Work out the finished part from the listing and answer in its coordinate system (mm). Face numbers are marked on the shaded views. Coordinates: 2 decimals unless noted, no trailing zeros. Order: outer loops, then holes, each group sorted by start corner. A loop starts at its lowest first (then second) coordinate and runs counter-clockwise, first axis right, second up. Notation, with made-up numbers: M 29.5,40.25 L 61.5,40.25 A20 cw 61.5,60.25 Z; hole C 40.5,54 d1. An arc over 180 degrees is marked long. Answer in a Markdown table with one row per item. Add a question column.
Item 1: Flat-ended cylindrical pins translate along their axes: pin 1 Ø3 at (x, y) = (42.5, 19.5) entering from +Z; pin 2 Ø1 at (x, z) = (43.5, -2) entering from -Y; pin 3 Ø1.6 at (y, z) = (32, -2) entering from +X; pin 4 Ø1 at (y, z) = (7.5, -0.5) entering from +X. Find the tip coordinate at first contact, or state that the pin passes through.
Item 2: Consider line 1 (Y direction, x = 12.7, z = -1.5); line 2 (Y direction, x = 14, z = -2.35); line 3 (X direction, y = 39.5, z = -0.75). Determine where each line is inside the solid, lowest interval first. Write a range as from..to.
Item 3: The part is cut by section B-B (y = 63.5). Write down the section's boundary in (x, z) (3 decimals).
Item 4: The part is cut by section C-C (y = 12.7). Write down the section's boundary in (x, z) (3 decimals), then the cut area to 3 significant figures.
Item 5: The mould has two halves that part along Z. Classify the marked faces 1 and 2: released by +Z, released by -Z, zero draft, split by the parting line, or undercut.
Item 6: The part is cut by section A-A (x = 63.5). Write down the section's boundary in (y, z) (3 decimals).
Item 7: The part is cut by section D-D (z = -1.1). Write down the section's boundary in (x, y).
from build123d import *

# Parameters (mm, degrees)
BOSS_EXTRUDE1_DEPTH = 3.175
SKETCH2_R           = 2.4892
CUT_EXTRUDE1_DEPTH  = 108.809835474
FILLET3_R           = 2.54


with BuildPart() as part:
    # Sketch1 → Boss-Extrude1 (new body)
    with BuildSketch(Plane.XY):
        Polygon((25.4, 0), (0, 0), (0, 76.2), (76.2, 76.2), (76.2, 50.8), align=None)
        Polygon((58.239487758, 50.8), (25.4, 50.8), (25.4, 17.960512242), align=None, mode=Mode.SUBTRACT)
    extrude(amount=-BOSS_EXTRUDE1_DEPTH)

    # Sketch2 → Cut-Extrude1 (cut, through all)
    with BuildSketch(Plane.XY):
        with Locations((12.7, 63.5)):
            Circle(SKETCH2_R)
        with Locations((38.1, 63.5)):
            Circle(SKETCH2_R)
        with Locations((63.5, 63.5)):
            Circle(SKETCH2_R)
        with Locations((12.7, 38.1)):
            Circle(SKETCH2_R)
        with Locations((12.7, 12.7)):
            Circle(SKETCH2_R)
    extrude(amount=-CUT_EXTRUDE1_DEPTH, mode=Mode.SUBTRACT)

    # Fillet3
    fillet3_edges = [part.edges().sort_by_distance(p)[0] for p in [
        (25.4, 50.8, -1.5875),
        (25.4, 17.960512242, -1.5875),
        (58.239487758, 50.8, -1.5875),
        (0, 0, -1.5875),
        (0, 76.2, -1.5875),
        (76.2, 76.2, -1.5875),
        (76.2, 50.8, -1.5875),
        (25.4, 0, -1.5875),
    ]]
    fillet(fillet3_edges, radius=FILLET3_R)


solid = part.part
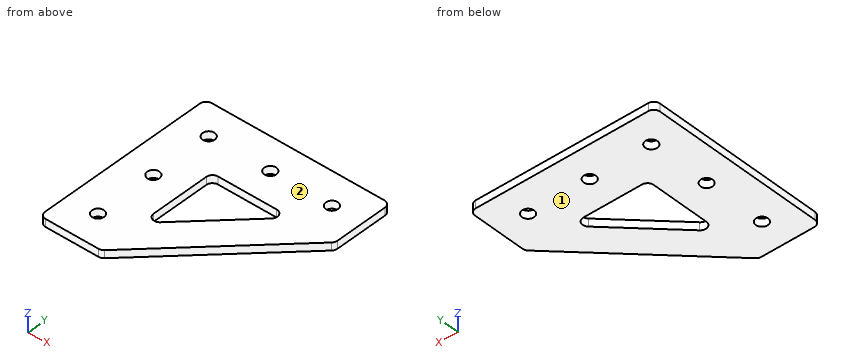
Reply:
| question | item | result |
|---|---|---|
| 1 | pin 1 | stops at z = 0 |
| 1 | pin 2 | stops at y = 17.6 |
| 1 | pin 3 | stops at x = 58.2 |
| 1 | pin 4 | stops at x = 33.4 |
| 2 | line 1 | y = 0..10.21, 15.19..35.61, 40.59..61.01, 65.99..76.2 |
| 2 | line 2 | y = 0..10.58, 14.82..35.98, 40.22..61.38, 65.62..76.2 |
| 2 | line 3 | x = 0..10.64, 14.76..25.4, 46.94..64.9 |
| 3 | outline | M 0,-3.175 L 10.211,-3.175 L 10.211,0 L 0,0 Z; M 15.189,-3.175 L 35.611,-3.175 L 35.611,0 L 15.189,0 Z; M 40.589,-3.175 L 61.011,-3.175 L 61.011,0 L 40.589,0 Z; M 65.989,-3.175 L 76.2,-3.175 L 76.2,0 L 65.989,0 Z |
| 4 | outline | M 0,-3.175 L 10.211,-3.175 L 10.211,0 L 0,0 Z; M 15.189,-3.175 L 38.1,-3.175 L 38.1,0 L 15.189,0 Z |
| 4 | area | 105 mm2 |
| 5 | face 1 | released by -Z |
| 5 | face 2 | released by +Z |
| 6 | outline | M 38.1,-3.175 L 61.011,-3.175 L 61.011,0 L 38.1,0 Z; M 65.989,-3.175 L 76.2,-3.175 L 76.2,0 L 65.989,0 Z |
| 7 | outline | M 0,2.54 A2.54 ccw 2.54,0 L 24.35,0 A2.54 ccw 26.14,0.74 L 75.46,50.06 A2.54 ccw 76.2,51.85 L 76.2,73.66 A2.54 ccw 73.66,76.2 L 2.54,76.2 A2.54 ccw 0,73.66 Z; hole C 12.7,12.7 d4.98; hole C 12.7,38.1 d4.98; hole C 12.7,63.5 d4.98; hole M 25.4,24.09 A2.54 ccw 29.74,22.3 L 53.9,46.46 A2.54 ccw 52.11,50.8 L 27.94,50.8 A2.54 ccw 25.4,48.26 Z; hole C 38.1,63.5 d4.98; hole C 63.5,63.5 d4.98 |
